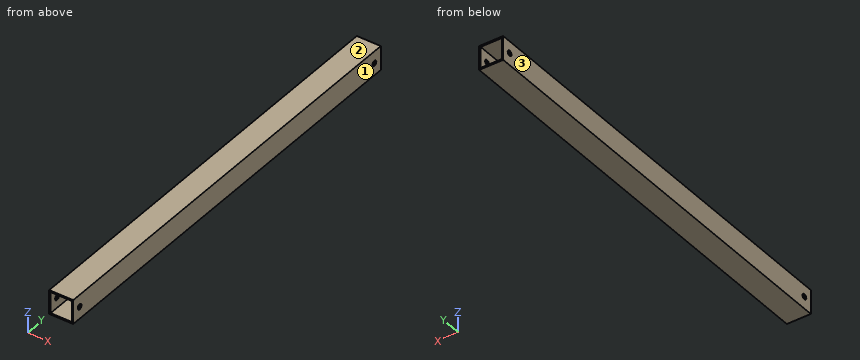
```python
from build123d import *

# Parameters (mm, degrees)
F0_W     = 25.4
F0_H     = 25.4
F0_W_2   = 22.352
F0_H_2   = 22.352
F1_DEPTH = 457.2
F2_R     = 2.778125
F3_DEPTH = 25.4
F4_R     = 2.778125
F5_DEPTH = 25.4


with BuildPart() as f1:
    # F0 (on Front) → F1 (new body)
    with BuildSketch(Plane.XZ):
        Rectangle(F0_W, F0_H)
        Rectangle(F0_W_2, F0_H_2, mode=Mode.SUBTRACT)
    extrude(amount=-F1_DEPTH)

    # F2 (on face) → F3 (cut)
    with BuildSketch(Plane.YZ.offset(12.7)):
        with Locations((9.525, 0)):
            Circle(F2_R)
    extrude(amount=-F3_DEPTH, mode=Mode.SUBTRACT)

    # F4 (on face) → F5 (cut)
    with BuildSketch(Plane.YZ.offset(12.7)):
        with Locations((447.675, 0)):
            Circle(F4_R)
    extrude(amount=-F5_DEPTH, mode=Mode.SUBTRACT)


solid = f1.part
```
CAD build for the part. Positions are in the model's coordinates, mm. Face numbers are marked on the shaded views. Give positions to 0.01 mm unless a question says otherwise; leave off trailing zeros. Order: outer loops, then holes, each group sorted by start corner. A loop starts at its lowest first (then second) coordinate and runs counter-clockwise, first axis right, second up. Notation, with made-up numbers: M 17.25,-37 L 45.25,-37 A37 cw 45.25,0 Z; hole C 17,65.5 d7. An arc over 180 degrees is marked long. Put each result on its own line as item: value. Start each with the question number.
(1) Saw through at A-A, the plane z = 7. Write the cut outline in (x, y), then the cut area to 3 significant figures.
(2) Mould opens along X. For the marked faces 1, 2 and 3 say: +X half, -X half, draft (parallel to the pull), parting line (faces both ways), or undercut.
(3) Saw through at C-C, the plane x = 2. Write the cut outline in (y, z), then the cut area to 3 significant figures.
(4) Saw through at B-B, the plane y = 333.5. Write the cut outline in (x, z).
(5) Drill centre lines: line 1 along Z through (x, y) = (2, 313.5); line 2 along Y through (x, z) = (-11.25, -1). Where is each one in solid material? Low to high.
Check result:
1. outline: M -12.7,0 L -11.18,0 L -11.18,457.2 L -12.7,457.2 Z; M 11.18,0 L 12.7,0 L 12.7,457.2 L 11.18,457.2 Z
1. area: 1,390 mm2
2. face 1: +X half
2. face 2: draft
2. face 3: -X half
3. outline: M 0,-12.7 L 457.2,-12.7 L 457.2,-11.18 L 0,-11.18 Z; M 0,11.18 L 457.2,11.18 L 457.2,12.7 L 0,12.7 Z
3. area: 1,390 mm2
4. outline: M -12.7,-12.7 L 12.7,-12.7 L 12.7,12.7 L -12.7,12.7 Z; hole M -11.18,-11.18 L 11.18,-11.18 L 11.18,11.18 L -11.18,11.18 Z
5. line 1: z = -12.7 to -11.18, 11.18 to 12.7
5. line 2: y = 0 to 6.93, 12.12 to 445.08, 450.27 to 457.2
